The model under review builds one solid part; all positions refer to its coordinate system, in mm. A direction names the side the tool comes from. Coordinates: 2 decimals unless noted, no trailing zeros. Order: outer loops, then holes, each group sorted by start corner. A loop starts at its lowest first (then second) coordinate and runs counter-clockwise, first axis right, second up. Notation, with made-up numbers: M 76.25,4.5 L 111.25,4.5 A13 cw 111.25,27.5 Z; hole C -24.75,42 d7. An arc over 180 degrees is marked long. Answer as CSV lines item,"result". Start each with the question number.
Q1. The part is to be moulded in two halves that separate along Z. For faces 4 (the face through (7, 2, -2.35)), 5 (the face through (0.01, -3.24, -14.69)), 6 (the face through (-0.96, -5.56, -20.29)), say which applies: +Z half, -Z half, draft (parallel to the pull), parting line (faces both ways), or undercut.
Q2. Wall thickness on L1, parallel to X at y = 1.2, z = 1.15; L2, parallel to X at y = -12, z = -24.5; L3, parallel to Z at x = 9.4, y = 3.1: over which ranges is each line inside the solid? List them lowest first. Write a range as [from, to].
Q3. Consider section D-D on x = 22.5. Write out the cut boundary in (y, z) (3 decimals).
Q4. Machinability: for faces 1 (the face through (0.8, -2, -16)), 2 (the face through (22, -13.45, -24)), 3 (the face through (-2, -16.8, -25)), which of the approach directions +Z, -Z, +X, -X, +Y, -Y give a long, thin tool a straight path to every point of the face, cutting with its end or side? Answer none if there is none.
Q5. Consider section B-B on y = -3. Write out the cut boundary in (x, z), and give its area (3 significant figures).
Q6. For P1, Ø2, axis at x = 5, z = -7, coming from the -Y side; P2, Ø14, axis at x = 5, z = -8.5, coming from the +Y side; P3, Ø2, axis at x = 12.5, y = -5.5, coming from the -Z side (3 decimals), all flat-tipped, find the tip position at first contact; note any pin that passes through.
Q7. Consider section C-C on y = 2. Write out the cut boundary in (x, z).
Q8. Consider section A-A on z = -12. Write out the cut boundary in (x, y), and give its area (3 significant figures).
from build123d import *
from build123d.topology import SkipClean

# Parameters (mm, degrees)
SKETCH2_R           = 1.4
SKETCH2_R_2         = 2.5
BOSS_EXTRUDE1_DEPTH = 4
BOSS_EXTRUDE2_START = 16.8
SKETCH3_R           = 4.65
SKETCH3_R_2         = 2.5
BOSS_EXTRUDE2_DEPTH = 16.8
SKETCH5_R           = 4.65
SKETCH5_R_2         = 2.5
BOSS_EXTRUDE3_DEPTH = 2
FILLET1_R           = 2
RIB1_REACH          = 36.514
SKETCH6_WALL_W      = 80.220281068
SKETCH6_WALL_H      = 1.6
BOSS_EXTRUDE4_DEPTH = 5.65
SKETCH8_R           = 3.125
BOSS_EXTRUDE5_DEPTH = 1.8
SKETCH9_R           = 1.4
CUT_EXTRUDE1_DEPTH  = 43.420130834
RIB2_REACH          = 43.272
SKETCH10_WALL_W     = 92.747093244
SKETCH10_WALL_H     = 1.7


with BuildPart() as part:
    # Sketch2 → Boss-Extrude1 (new body)
    with BuildSketch(Plane(origin=(0, 0, 0), x_dir=(1, 0, 0), z_dir=(0, 1, 0))):
        with BuildLine():
            Line((-9.4, -4.65), (0, -4.65))
            ThreePointArc((0, -4.65), (3.288046533, -3.288046533), (4.65, 0))
            Line((4.65, 0), (4.65, 22.6))
            ThreePointArc((4.65, 22.6), (0, 27.25), (-4.65, 22.6))
            Line((-4.65, 22.6), (-4.65, 2.35))
            Line((-4.65, 2.35), (-9.4, 2.35))
            ThreePointArc((-9.4, 2.35), (-12.9, -1.15), (-9.4, -4.65))
        make_face()
        with Locations(Location((-9.4, -1.15, 0), (0, 0, 270))):
            Circle(SKETCH2_R, mode=Mode.SUBTRACT)
        with Locations(Location((0, -1.15, 0), (0, 0, 270))):
            Circle(SKETCH2_R, mode=Mode.SUBTRACT)
        with Locations(Location((0, 22.6, 0), (0, 0, 270))):
            Circle(SKETCH2_R_2, mode=Mode.SUBTRACT)
    extrude(amount=BOSS_EXTRUDE1_DEPTH)

    # Sketch3 → Boss-Extrude2 (add)
    with BuildSketch(Plane.XZ.offset(BOSS_EXTRUDE2_START)):
        with Locations((0, -22.6)):
            Circle(SKETCH3_R)
        with Locations(Location((0, -22.6, 0), (0, 0, 90))):
            Circle(SKETCH3_R_2, mode=Mode.SUBTRACT)
    extrude(amount=-BOSS_EXTRUDE2_DEPTH)

    # Sketch5 → Boss-Extrude3 (add)
    with SkipClean():  # the faces are left unmerged after this step: merging them gives an invalid solid
        with BuildSketch(Plane(origin=(0, 4, 0), x_dir=(1, 0, 0), z_dir=(0, 1, 0))):
            with Locations(Location((0, 22.6, 0), (0, 0, 270))):
                Circle(SKETCH5_R)
            with Locations(Location((0, 22.6, 0), (0, 0, 270))):
                Circle(SKETCH5_R_2, mode=Mode.SUBTRACT)
        extrude(amount=BOSS_EXTRUDE3_DEPTH)

    # Fillet1
    fillet1_edges = [part.edges().sort_by_distance(p)[0] for p in [
        (0, 6, -27.25),
    ]]
    fillet(fillet1_edges, radius=FILLET1_R - 0.0001)  # a hair under: the kernel refuses the full size

    # Sketch6 wall → Rib1 (add, up to next)
    with BuildSketch(Plane(origin=(0, -3.25, -14.7), x_dir=(0, -0.707106781187, -0.707106781187), z_dir=(0, 0.707106781187, -0.707106781187)), mode=Mode.PRIVATE) as rib1_sk1:
        Rectangle(SKETCH6_WALL_W, SKETCH6_WALL_H)
    rib1_tool1 = extrude(rib1_sk1.sketch, amount=RIB1_REACH, mode=Mode.PRIVATE) - part.part
    add(rib1_tool1.solids().sort_by_distance((0, -3.25, -14.7))[0])


with BuildPart() as body_2:
    # Mirror1: mirrored copy
    add(part.part.mirror(Plane(origin=(0, 0, 0), x_dir=(0, 0, 1), z_dir=(1, 0, 0))))

    # Sketch7 → Boss-Extrude4 (add)
    with BuildSketch(Plane(origin=(0, -6, 0), x_dir=(1, 0, 0), z_dir=(0, 1, 0))):
        with BuildLine():
            Line((22.925, 25.725), (3.443381332, 25.725))
            ThreePointArc((3.443381332, 25.725), (4.65, 22.6), (3.443381332, 19.475))
            Line((3.443381332, 19.475), (22.925, 19.475))
            ThreePointArc((22.925, 19.475), (26.05, 22.6), (22.925, 25.725))
        make_face()
    extrude(amount=-BOSS_EXTRUDE4_DEPTH)

    # Sketch8 → Boss-Extrude5 (add)
    with SkipClean():  # the faces are left unmerged after this step: merging them gives an invalid solid
        with BuildSketch(Plane.XZ.offset(11.65)):
            with Locations(Location((22.925, -22.6, 0), (0, 0, 270))):
                Circle(SKETCH8_R)
        extrude(amount=BOSS_EXTRUDE5_DEPTH)
    add(body_2.part.scale(1), mode=Mode.REPLACE)  # the faces are merged on a copy

    # Sketch9 → Cut-Extrude1 (cut, through all)
    with BuildSketch(Plane.XZ.offset(13.45)):
        with Locations(Location((22.925, -22.6, 0), (0, 0, 270))):
            Circle(SKETCH9_R)
    extrude(amount=-CUT_EXTRUDE1_DEPTH, mode=Mode.SUBTRACT)

    # Sketch10 wall → Rib2 (add, up to next)
    with BuildSketch(Plane(origin=(7.55, -3.1, -22.6), x_dir=(0.707106781187, -0.707106781187, 0), z_dir=(0.707106781187, 0.707106781187, 0)), mode=Mode.PRIVATE) as rib2_sk1:
        Rectangle(SKETCH10_WALL_W, SKETCH10_WALL_H)
    rib2_tool1 = extrude(rib2_sk1.sketch, amount=-RIB2_REACH, mode=Mode.PRIVATE) - body_2.part
    add(rib2_tool1.solids().sort_by_distance((7.55, -3.1, -22.6))[0])


solid = body_2.part
Evaluation:
1,face 4,"-Z half"
1,face 5,"+Z half"
1,face 6,"undercut"
2,L1,"x = [-4.51, -1.4], [1.4, 8], [10.8, 12.9]"
2,L2,"x = [-4.24, -1.62], [1.62, 4.24], [20.44, 25.41]"
2,L3,"z = [-2.35, -0.25], [2.55, 4.65]"
3,outline,"M -13.45,-25.696 L -11.65,-25.696 L -11.65,-25.725 L -6,-25.725 L -6,-23.934 L -13.45,-23.934 Z; M -13.45,-21.266 L -6,-21.266 L -6,-19.475 L -11.65,-19.475 L -11.65,-19.504 L -13.45,-19.504 Z"
4,face 1,"+Z, +X, -Y"
4,face 2,"+Z, -Z, +X, -Y"
4,face 3,"+Z, -Z, +X, -X, -Y"
5,outline,"M -0.8,-18.02 A4.65 ccw long 4.57,-23.45 L 7.45,-23.45 L 7.45,-21.75 L 4.57,-21.75 A4.65 ccw 0.8,-18.02 L 0.8,-14.45 L -0.8,-14.45 Z; hole C 0,-22.6 d5"
5,area,"58.7 mm²"
6,P1,"stops at y = 0"
6,P2,"stops at y = 4"
6,P3,"stops at z = -25.725"
7,outline,"M -4.65,-22.6 A4.65 ccw 4.65,-22.6 L 4.65,-2.35 L 9.4,-2.35 A3.5 ccw 9.4,4.65 L 0,4.65 A4.65 ccw -4.65,0 Z; hole C 0,-22.6 d5; hole C 0,1.15 d2.8; hole C 9.4,1.15 d2.8"
8,outline,"M -4.65,0 L -0.8,0 L -0.8,-0.55 L 0.8,-0.55 L 0.8,0 L 4.65,0 L 4.65,4 L -4.65,4 Z"
8,area,"38.1 mm²"
